The listing builds one solid part. Answer for the finished solid, in the listing's coordinates (mm). Face numbers are marked on the shaded views. A direction names the side the tool comes from. Round coordinates to 2 decimals unless told otherwise and drop trailing zeros. Loops run counter-clockwise (first coordinate to the right, second up) from the corner with the lowest first, then second, coordinate; pieces in that order, holes last. Notation, with made-up numbers: (53, 21.25) - (67, 21.25) arc R23 ccw to (67, 50.25) - close; hole circle Ø9 at (-12.75, -37). An arc over 180 degrees is marked (long way). Write item = value, one per line. Start each with the question number.
1) Straight lines are drawn through the part: line 1 along Y through (x, z) = (0, -2.75); line 2 along Y through (x, z) = (5, -0.75); line 3 along X through (y, z) = (2.75, -0.5). For each, find the intervals that lie inside material, in ascending order.
2) Section A-A, the plane z = -2.5 is taken. Determine the outline of the cut face in (x, y), and give its area (3 significant figures).
3) A tool of negligible diameter and unlimited length cuts with its end or side. For the marked faces 1, 2 and 3, from which of +Z, -Z, +X, -X, +Y, -Y can it reach the whole face along a straight path? Write none if from no direction.
4) Section B-B, the plane x = 3 is taken. Determine the outline of the cut face in (y, z).
5) Section C-C, the plane y = -2 is taken. Determine the outline of the cut face in (x, z), and give its area (3 significant figures).
6) For a pull along X with two mould halves and no side action, classify the marked faces 4, 5, 6 and 7 as released by +X, released by -X, zero draft, split by the parting line, or undercut.
7) Section D-D, the plane z = -7.5 is taken. Determine the outline of the cut face in (x, y), and give its area (3 significant figures).
8) Given pin 1 Ø6 at (y, z) = (6, -8.5) entering from +X; pin 2 Ø5 at (x, y) = (-10.5, 0) entering from -Z, each flat-ended and moving along its own axis, determine where each tip first touches the part or whether it passes through.
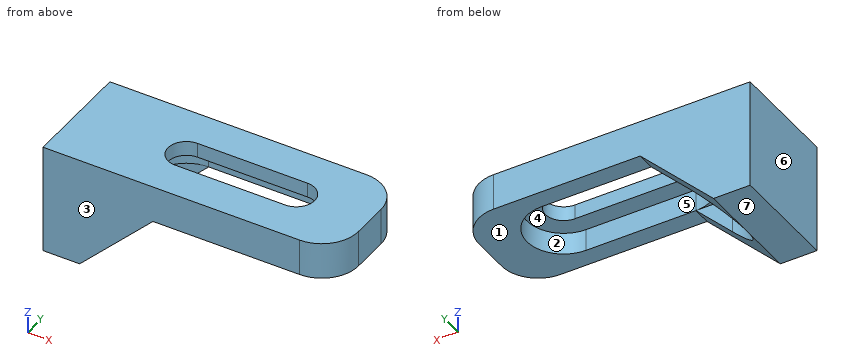
from build123d import *

# Parameters (mm, degrees)
EXTRUDE_1_DEPTH     = 2
EXTRUDE_2_DEPTH     = 5
EXTRUDE_3_DEPTH     = 15
EXTRUDE_4_DEPTH     = 15
CUT_EXTRUDE_START   = -5
CUT_EXTRUDE_1_DEPTH = 15


with BuildPart() as part:
    # Sketch 1 → Extrude 1 (new body)
    with BuildSketch(Plane.XY):
        with BuildLine():
            Line((-20, -7.5), (15, -7.5))
            ThreePointArc((15, -7.5), (18.535533906, -6.035533906), (20, -2.5))
            Line((20, -2.5), (20, 2.5))
            ThreePointArc((20, 2.5), (18.535533906, 6.035533906), (15, 7.5))
            Line((15, 7.5), (-20, 7.5))
            Line((-20, 7.5), (-20, -7.5))
        make_face()
        with BuildLine():
            Line((-5, 2.5), (10, 2.5))
            ThreePointArc((10, 2.5), (12.5, 0), (10, -2.5))
            Line((10, -2.5), (-5, -2.5))
            ThreePointArc((-5, -2.5), (-7.5, 0), (-5, 2.5))
        make_face(mode=Mode.SUBTRACT)
    extrude(amount=-EXTRUDE_1_DEPTH)

    # Sketch 1_3 → Extrude 2 (add)
    with BuildSketch(Plane.XY):
        with BuildLine():
            Line((15, 7.5), (-20, 7.5))
            Line((-20, 7.5), (-20, -7.5))
            Line((-20, -7.5), (15, -7.5))
            ThreePointArc((15, -7.5), (18.535533906, -6.035533906), (20, -2.5))
            Line((20, -2.5), (20, 2.5))
            ThreePointArc((20, 2.5), (18.535533906, 6.035533906), (15, 7.5))
        make_face()
        with BuildLine():
            ThreePointArc((-5, -5), (-10, 0), (-5, 5))
            Line((-5, 5), (10, 5))
            ThreePointArc((10, 5), (15, 0), (10, -5))
            Line((10, -5), (-5, -5))
        make_face(mode=Mode.SUBTRACT)
    extrude(amount=-EXTRUDE_2_DEPTH)

    # Sketch 1_4 → Extrude 3 (add)
    with BuildSketch(Plane.XY):
        Polygon((-15, 0), (-15, 7.5), (-20, 7.5), (-20, -7.5), (-15, -7.5), align=None)
    extrude(amount=-EXTRUDE_3_DEPTH)

    # Sketch 2 → Extrude 4 (add)
    with BuildSketch(Plane(origin=(0, 7.5, 0), x_dir=(1, 0, 0), z_dir=(0, 1, 0))):
        Polygon((-15, 15), (-5, 5), (-15, 5), align=None)
    extrude(amount=-EXTRUDE_4_DEPTH)

    # Sketch 1_5 → Cut-Extrude 1 (cut)
    with BuildSketch(Plane.XY.offset(CUT_EXTRUDE_START)):
        with BuildLine():
            Line((-10, 5), (10, 5))
            ThreePointArc((10, 5), (15, 0), (10, -5))
            Line((10, -5), (-10, -5))
            ThreePointArc((-10, -5), (-15, 0), (-10, 5))
        make_face()
    extrude(amount=-CUT_EXTRUDE_1_DEPTH, mode=Mode.SUBTRACT)


solid = part.part
Geometry check:
q1.line_1 = -7.5 to -5, 5 to 7.5
q1.line_2 = -7.5 to -2.5, 2.5 to 7.5
q1.line_3 = -20 to 19.99
q2.outline = (-20, -7.5) - (15, -7.5) arc R5 ccw to (20, -2.5) - (20, 2.5) arc R5 ccw to (15, 7.5) - (-20, 7.5) - close; hole (-5, -5) - (10, -5) arc R5 ccw to (10, 5) - (-5, 5) arc R5 ccw to start
q2.area = 361 mm2
q3.face_1 = -Z, +X, +Y, -Y
q3.face_2 = -Z
q3.face_3 = +Z, -Z, +X, -X, -Y
q4.outline = (-7.5, -5) - (-5, -5) - (-5, -2) - (-2.5, -2) - (-2.5, 0) - (-7.5, 0) - close; (2.5, -2) - (5, -2) - (5, -5) - (7.5, -5) - (7.5, 0) - (2.5, 0) - close
q5.outline = (-20, -15) - (-15, -15) - (-14.58, -14.58) - (-14.58, -5) - (-9.58, -5) - (-9.58, -2) - (-6.5, -2) - (-6.5, 0) - (-20, 0) - close; (11.5, -2) - (14.58, -2) - (14.58, -5) - (20, -5) - (20, 0) - (11.5, 0) - close
q5.area = 146 mm2
q6.face_4 = undercut
q6.face_5 = undercut
q6.face_6 = released by -X
q6.face_7 = zero draft
q7.outline = (-20, -7.5) - (-7.5, -7.5) - (-7.5, -5) - (-10, -5) arc R5 cw to (-10, 5) - (-7.5, 5) - (-7.5, 7.5) - (-20, 7.5) - close
q7.area = 123 mm2
q8.pin_1 = -5.5
q8.pin_2 = -5
